Part model, mm, in its own coordinate system. A direction names the side the tool comes from. Coordinates: 2 decimals unless noted, no trailing zeros. Loops run counter-clockwise (first coordinate to the right, second up) from the corner with the lowest first, then second, coordinate; pieces in that order, holes last. Notation, with made-up numbers: M 65,8 L 77,8 A27 cw 77,26 Z; hole C -3.5,34.25 d11. An arc over 180 degrees is marked long. Answer as a JSON object with one key per item and string values. Group by question number.
1. Drill centre lines: L1, parallel to Z at x = 4.75, y = -5.5; L2, parallel to Z at x = 8.5, y = 5; L3, parallel to X at y = 1.5, z = 6. Where is each one in solid material? Low to high.
2. Mould opens along Y. For faces 3 (the face through (5.152, 2.832, -7.048)), 4 (the face through (-2.44, -1.809, -5.745)), 5 (the face through (0, -2, -7)) say: released by +Y, released by -Y, zero draft, split by the parting line, or undercut.
3. Saw through at C-C on x = -1.75. Write the cut outline in (y, z), then the cut area to 3 significant figures.
4. Saw through at B-B on y = 7. Write the cut outline in (x, z).
5. Saw through at A-A on z = -7.5. Write the cut outline in (x, y).
6. Drop flat-ended pins along their axis: pin 1 Ø2.5 at (y, z) = (7.5, -2) entering from -X; pin 2 Ø3 at (x, z) = (3.5, 5) entering from +Y. Give the stop position or say it passes through.
7. 3-axis set-ups, long thin cutter, end or side, ignore diameter. For faces 1 (the face through (-4.95, 3.92, -1.42)), 2 (the face through (0, 5, 5)): which of +Z, -Z, +X, -X, +Y, -Y reach the whole face in a straight line?
from build123d import *

# Parameters (mm, degrees)
BASPROSKE_W             = 12.7
BASPROSKE_H             = 8.89
TOOTHCUT_DEPTH          = 18.870484045
TEETHCUTS_COUNT         = 12
TEETHCUTS_ANGLE         = 330
BORSKE_R                = 3
BORE_DEPTH              = 50.8000508
SKETCH2_W               = 2.25
SKETCH2_H               = 17.280564042
CUT_EXTRUDE1_DEPTH      = 18.6238176
CUT_EXTRUDE1_DEPTH_BACK = 18.6238176


with BuildPart() as part:
    # BasProSke → Base-Revolve (revolve)
    with BuildSketch(Plane(origin=(0, 0, 0), x_dir=(1, 0, 0), z_dir=(0, 1, 0)), mode=Mode.PRIVATE) as base_revolve_sk:
        with Locations((6.35, 4.445)):
            Rectangle(BASPROSKE_W, BASPROSKE_H)
    revolve(base_revolve_sk.sketch.rotate(Axis((-10, 0, 0), (1, 0, 0)), 180), axis=Axis((-10, 0, 0), (1, 0, 0)))

    # TooCutSke → ToothCut (cut, through all)
    with BuildSketch(Plane(origin=(0, 0, 0), x_dir=(0, 0, -1), z_dir=(1, 0, 0))):
        with BuildLine():
            ThreePointArc((0.717076553, 6.002519826), (0, 6.0452), (-0.717076553, 6.002519826))
            ThreePointArc((-0.717076553, 6.002519826), (-1.069160545, 7.516029346), (-2.121611652, 8.659279483))
            ThreePointArc((-2.121611652, 8.659279483), (0, 8.9154), (2.121611652, 8.659279483))
            ThreePointArc((2.121611652, 8.659279483), (1.069160545, 7.516029346), (0.717076553, 6.002519826))
        make_face()
    toothcut = extrude(amount=TOOTHCUT_DEPTH, mode=Mode.SUBTRACT)

    # TeethCuts: ToothCut ×12 about axis
    teethcuts_axis = Axis((-10, 0, 0), (1, 0, 0))
    for i in range(1, TEETHCUTS_COUNT):
        add(toothcut.rotate(teethcuts_axis, i * TEETHCUTS_ANGLE / (TEETHCUTS_COUNT - 1)), mode=Mode.SUBTRACT)

    # BorSke → Bore (cut, symmetric)
    with BuildSketch(Plane(origin=(0, 0, 0), x_dir=(0, 0, -1), z_dir=(1, 0, 0))):
        with Locations(Location((0, 0, 0), (0, 0, 180))):
            Circle(BORSKE_R)
    extrude(amount=BORE_DEPTH, both=True, mode=Mode.SUBTRACT)

    # Sketch1 → Revolve1 (revolve)
    with BuildSketch(Plane.XY, mode=Mode.PRIVATE) as revolve1_sk:
        Polygon((0, -4), (-4.95, -4), (-4.95, -6), (0, -6.0452), align=None)
    revolve(revolve1_sk.sketch.rotate(Axis((0, 0, 0), (-1, 0, 0)), 270), axis=Axis((0, 0, 0), (-1, 0, 0)))

    # Sketch2 → Cut-Extrude1 (cut, two sides)
    with BuildSketch(Plane.XY) as cut_extrude1_sk:
        with Locations((11.575, 0)):
            Rectangle(SKETCH2_W, SKETCH2_H)
    extrude(amount=CUT_EXTRUDE1_DEPTH, mode=Mode.SUBTRACT)
    extrude(cut_extrude1_sk.sketch, amount=-CUT_EXTRUDE1_DEPTH_BACK, mode=Mode.SUBTRACT)


solid = part.part
Outcome:
{
 "1": {"L1": "z = -6.33 to -4.1, -2.51 to 2.51, 4.1 to 6.33", "L2": "z = -6.15 to -3.72, -3.4 to 3.4, 3.72 to 6.15", "L3": "x = 0 to 10.45"},
 "2": {"face 3": "undercut", "face 4": "split by the parting line", "face 5": "zero draft"},
 "3": {"outline": "C 0,0 d12.06; hole C 0,0 d8", "area": "63.9 mm²"},
 "4": {"outline": "M 0,-2.83 L 10.45,-2.83 L 10.45,-0.85 L 0,-0.85 Z; M 0,0.85 L 10.45,0.85 L 10.45,2.83 L 0,2.83 Z"},
 "5": {"outline": "M 0,-2.81 L 10.45,-2.81 L 10.45,-1.06 L 0,-1.06 Z; M 0,1.06 L 10.45,1.06 L 10.45,2.81 L 0,2.81 Z"},
 "6": {"pin 1": "stops at x = 0", "pin 2": "stops at y = 6.44"},
 "7": {"face 1": "+Z, -Z, -X, +Y, -Y", "face 2": "+Z, -X, +Y"}
}
